Input: part model. Units: mm. Frame: model coordinates. A direction names the side the tool comes from. Round coordinates to 2 decimals unless told otherwise and drop trailing zeros. Order: outer loops, then holes, each group sorted by start corner. A loop starts at its lowest first (then second) coordinate and runs counter-clockwise, first axis right, second up.
Item 1: Cut plane A-A on x = 36.5. Output: boundary loops of the cut face in (y, z), then the cut area to 3 significant figures.
Item 2: Line query: L1, parallel to Z at x = 32.5, y = 112; L2, parallel to Y at x = 40, z = 1381.5; L3, parallel to Z at x = 8.5, y = 175.5. Output: solid intervals per line, ascending.
Item 3: First-contact query: pin 1 (10 mm diameter, centred on x = -1, z = 1388.5, fed in from -Y); pin 2 (1 mm diameter, centred on x = -28.5, z = 1397.5, fed in from +Y); pin 3 (1.5 mm diameter, centred on x = -2, y = 102, fed in from +Z); pin 4 (6.5 mm diameter, centred on y = 184, z = 1404, fed in from +X). Flat tips, straight axial feed; report the tip coordinate or a pass-through.
Item 4: Mould query, pull axis Y, two halves, no side actions, for faces 5 (the flat face through (2.93, 133.08, 1373.84)), 6 (the cylindrical face through (-17.21, 76.865, 1337.489)), 7 (the flat face through (29, 177, 1408)), 8 (the cylindrical face through (-17.21, 188.024, 1415.323)). Classes: released by +Y, released by -Y, zero draft, split by the parting line, or undercut.
Item 5: Reachability of faces 1 (the flat face through (-29.605, 97.357, 1351.838)), 2 (the flat face through (-29.605, 164.266, 1398.688)), 3 (the flat face through (36.395, 97.357, 1351.838)), 4 (the flat face through (36.395, 164.266, 1398.688)) from +Z, -Z, +X, -X, +Y, -Y: full face, straight path, thin tool, end or side. Return the list, or none.
Item 6: Cut plane B-B on z = 1343. Output: boundary loops of the cut face in (x, y).
```python
from build123d import *

# Parameters (mm, degrees)
CYLINDER083_R     = 2
CYLINDER083_DEPTH = 10
ARRAY001_X_COUNT  = 2
ARRAY001_X_PITCH  = 40.9
ARRAY001_Y_COUNT  = 2
ARRAY001_Y_PITCH  = 135.7
BOX080_W          = 51
BOX080_H          = 145.7
BOX080_DEPTH      = 5
BOX079_W          = 81
BOX079_H          = 81.68
BOX079_DEPTH      = 5
CUT086_ROLL_ANGLE = 35


with BuildPart() as array001:
    # Cylinder083 → Cylinder083 (new body)
    with BuildSketch(Plane(origin=(20.55, -5, 0), x_dir=(1, 0, 0), z_dir=(0, 0, 1))):
        Circle(CYLINDER083_R)
    extrude(amount=CYLINDER083_DEPTH)

    # Array001 X: Array001 ×2


with BuildPart() as array001_1:
    add(array001.part)
    with Locations(*[(i * ARRAY001_X_PITCH, 0, 0) for i in range(1, ARRAY001_X_COUNT)]):
        add(array001.part)

    # Array001 Y: Array001 ×2


with BuildPart() as array001_2:
    add(array001_1.part)
    with Locations(*[(0, i * ARRAY001_Y_PITCH, 0) for i in range(1, ARRAY001_Y_COUNT)]):
        add(array001_1.part)


with BuildPart() as array001_3:
    # Array001 placement: moved
    add(array001_2.part.moved(Location((0, 0, -2))))


with BuildPart() as cube028:
    # Box080 → Box080 (new body)
    with BuildSketch(Plane(origin=(15.5, -9.9875, 0), x_dir=(1, 0, 0), z_dir=(0, 0, 1))):
        with Locations((25.5, 72.85)):
            Rectangle(BOX080_W, BOX080_H)
    extrude(amount=BOX080_DEPTH)


with BuildPart() as tablet_holder_plate:
    # Box079 → Box079 (new body)
    with BuildSketch(Plane(origin=(0.5, 22, 0), x_dir=(1, 0, 0), z_dir=(0, 0, 1))):
        with Locations((40.5, 40.84)):
            Rectangle(BOX079_W, BOX079_H)
    extrude(amount=BOX079_DEPTH)

    # Fusion138: union Cube028
    add(cube028.part)

    # Cut086: cut Array001
    add(array001_3.part, mode=Mode.SUBTRACT)


with BuildPart() as tablet_holder_plate_1:
    # Cut086 roll: moved
    add(tablet_holder_plate.part.rotate(Axis((0, 0, 0), (1, 0, 0)), CUT086_ROLL_ANGLE))


with BuildPart() as tablet_holder_plate_2:
    # Cut086 placement: moved
    add(tablet_holder_plate_1.part.moved(Location((-37.5, 80.75, 1337.2))))


solid = tablet_holder_plate_2.part
```
From the geometry:
1. outline: (95.9, 1353.91) - (98.77, 1349.82) - (165.68, 1396.67) - (162.81, 1400.76) - close
1. area: 408 mm2
2. L1: z = 1359.08 to 1365.19
2. L2: y = 135.3 to 144.02
2. L3: z = 1403.54 to 1409.65
3. pin 1: stops at y = 138.16
3. pin 2: stops at y = 165.45
3. pin 3: stops at z = 1358.71
3. pin 4: passes through
4. face 5: released by +Y
4. face 6: undercut
4. face 7: zero draft
4. face 8: undercut
5. face 1: -Z, -X, -Y
5. face 2: +Z, -X, +Y
5. face 3: -Z, +X, -Y
5. face 4: +Z, +X, +Y
6. outline: (-22, 80.32) - (29, 80.32) - (29, 89.03) - (-22, 89.03) - close
